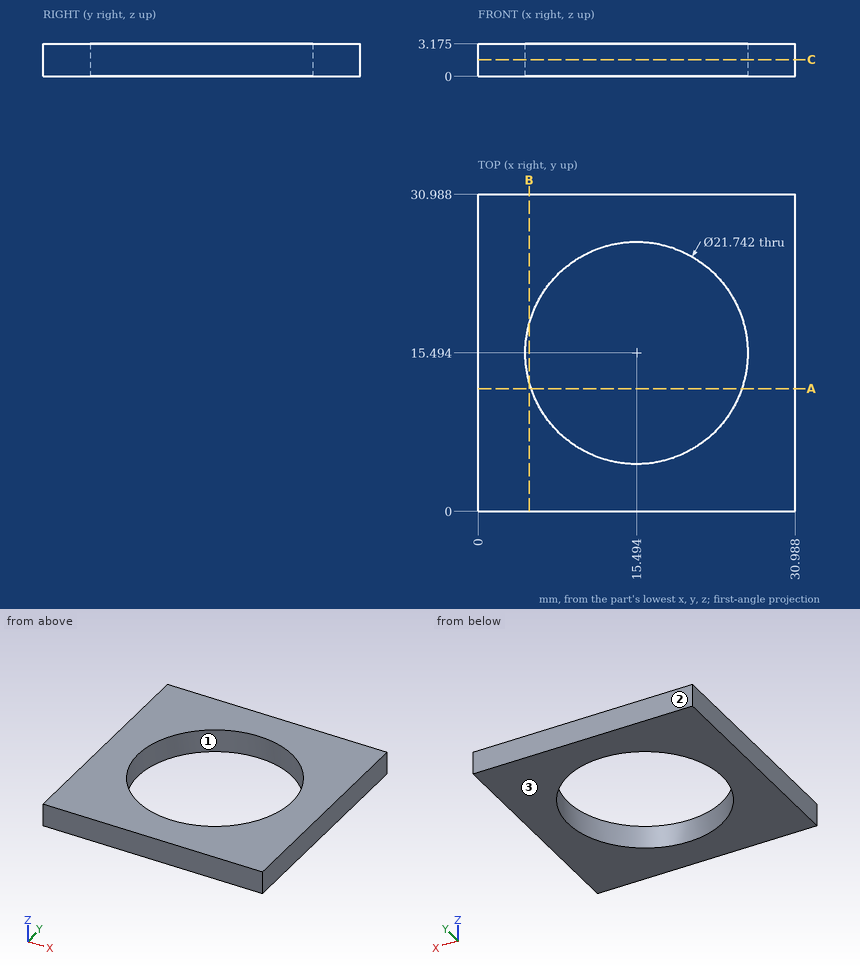
Geometry: see drawing. Coordinates: mm, zero at the bounding-box minimum. Round coordinates to 2 decimals unless told otherwise and drop trailing zeros. Write each loop counter-clockwise with the first axis right and the second up, starting at its lowest first coordinate (ties: lowest second). Pieces come first, ordered by that corner, then holes.
Item 1: Section query A-A (y = 12). Return loops of the section in (x, z) (1 decimal).
Item 2: Mould query, pull axis Y, two halves, no side actions, for the marked faces 1, 2 and 3. Classes: +Y half, -Y half, draft (parallel to the pull), parting line (faces both ways), or undercut.
Item 3: Pin query (flat end, axial travel): P1, Ø1.5, axis at x = 26.5, y = 25, coming from the -Z side; P2, Ø13, axis at x = 15.494, y = 15.494, coming from the +Z side (1 decimal). Return the tip coordinate at first contact, or that it passes through.
Item 4: Material intervals for L1, parallel to X at y = 19, z = 0.9 (1 decimal); L2, parallel to X at y = 16.5, z = 1.2; L3, parallel to Y at x = 12, z = 1.15, sorted ascending.
Item 5: Section query C-C (z = 1.65). Return loops of the section in (x, y), plus the area to 3 significant figures.
Item 6: Section query B-B (x = 5). Return loops of the section in (y, z) (1 decimal).
Completed:
1. outline: (0, 0) - (5.2, 0) - (5.2, 3.2) - (0, 3.2) - close; (25.8, 0) - (31, 0) - (31, 3.2) - (25.8, 3.2) - close
2. face 1: undercut
2. face 2: +Y half
2. face 3: draft
3. P1: stops at z = 0
3. P2: passes through
4. L1: x = 0 to 5.2, 25.8 to 31
4. L2: x = 0 to 4.67, 26.32 to 30.99
4. L3: y = 0 to 5.2, 25.79 to 30.99
5. outline: (0, 0) - (30.99, 0) - (30.99, 30.99) - (0, 30.99) - close; hole circle Ø21.74 at (15.49, 15.49)
5. area: 589 mm2
6. outline: (0, 0) - (12.7, 0) - (12.7, 3.2) - (0, 3.2) - close; (18.3, 0) - (31, 0) - (31, 3.2) - (18.3, 3.2) - close
